The listing builds one solid part. Answer for the finished solid, in the listing's coordinates (mm). A direction names the side the tool comes from. Give positions to 0.01 mm unless a question says otherwise; leave off trailing zeros. Order: outer loops, then holes, each group sorted by start corner. A loop starts at its lowest first (then second) coordinate and runs counter-clockwise, first axis right, second up. Notation, with made-up numbers: (5.5, 69) - (48.5, 69) arc R14 cw to (48.5, 82) - close; hole circle Ø8 at (-38.75, 33.25). An arc over 180 degrees is marked (long way). Answer in a Markdown table with one row per item. Add a question column.
```python
from build123d import *

# Parameters (mm, degrees)
SKETCH2_W           = 165
SKETCH2_H           = 140
SKETCH2_W_2         = 3
SKETCH2_H_2         = 146.3
SKETCH2_W_3         = 2.5
BOSS_EXTRUDE1_DEPTH = 5
SKETCH2_3_R         = 1.7
BOSS_EXTRUDE2_DEPTH = 2.5
SKETCH2_5_R         = 4
SKETCH2_5_R_2       = 1.7
BOSS_EXTRUDE3_DEPTH = 3
FILLET1_R           = 2


with BuildPart() as part:
    # Sketch2 → Boss-Extrude1 (new body)
    with BuildSketch(Plane(origin=(0, 0, 0), x_dir=(1, 0, 0), z_dir=(0, 1, 0))):
        Polygon((-88.5, -80), (-92.5, -80), (-92.5, -78.85), (-95.5, -78.85), (-95.5, -82.5), (95, -82.5), (95, -78.85), (92.5, -78.85), (92.5, -80), (88.5, -80), align=None)
        with BuildLine():
            Line((-92.5, -78.85), (-92.5, -80))
            Line((-92.5, -80), (-88.5, -80))
            ThreePointArc((-88.5, -80), (-90.016575089, -79.701351105), (-91.30668844, -78.85))
            Line((-91.30668844, -78.85), (-92.5, -78.85))
        make_face()
        with BuildLine():
            ThreePointArc((-91.30668844, -78.85), (-90.016575089, -79.701351105), (-88.5, -80))
            ThreePointArc((-88.5, -80), (-85.671572875, -78.828427125), (-84.5, -76))
            ThreePointArc((-84.5, -76), (-86.955130064, -72.310369005), (-91.30668844, -73.15))
            Line((-91.30668844, -73.15), (-90.145448267, -73.15))
            Line((-90.145448267, -73.15), (-86.854551733, -73.15))
            Line((-86.854551733, -73.15), (-85.209103466, -76))
            Line((-85.209103466, -76), (-86.854551733, -78.85))
            Line((-86.854551733, -78.85), (-90.145448267, -78.85))
            Line((-90.145448267, -78.85), (-91.30668844, -78.85))
        make_face()
        with BuildLine():
            ThreePointArc((-84.5, -76), (-85.671572875, -78.828427125), (-88.5, -80))
            Line((-88.5, -80), (88.5, -80))
            ThreePointArc((88.5, -80), (84.798648895, -74.483424911), (91.30668844, -73.15))
            Line((91.30668844, -73.15), (92.5, -73.15))
            Line((92.5, -73.15), (92.5, 73.15))
            Line((92.5, 73.15), (91.30668844, 73.15))
            ThreePointArc((91.30668844, 73.15), (84.798648895, 74.483424911), (88.5, 80))
            Line((88.5, 80), (-88.5, 80))
            ThreePointArc((-88.5, 80), (-85.671572875, 78.828427125), (-84.5, 76))
            ThreePointArc((-84.5, 76), (-86.955130064, 72.310369005), (-91.30668844, 73.15))
            Line((-91.30668844, 73.15), (-92.5, 73.15))
            Line((-92.5, 73.15), (-92.5, -73.15))
            Line((-92.5, -73.15), (-91.30668844, -73.15))
            ThreePointArc((-91.30668844, -73.15), (-86.955130064, -72.310369005), (-84.5, -76))
        make_face()
        Rectangle(SKETCH2_W, SKETCH2_H, mode=Mode.SUBTRACT)
        with Locations((-94, 0)):
            Rectangle(SKETCH2_W_2, SKETCH2_H_2)
        with BuildLine():
            Line((-92.5, 80), (-92.5, 78.85))
            Line((-92.5, 78.85), (-91.30668844, 78.85))
            ThreePointArc((-91.30668844, 78.85), (-90.016575089, 79.701351105), (-88.5, 80))
            Line((-88.5, 80), (-92.5, 80))
        make_face()
        with BuildLine():
            Line((-90.145448267, 73.15), (-91.30668844, 73.15))
            ThreePointArc((-91.30668844, 73.15), (-86.955130064, 72.310369005), (-84.5, 76))
            ThreePointArc((-84.5, 76), (-85.671572875, 78.828427125), (-88.5, 80))
            ThreePointArc((-88.5, 80), (-90.016575089, 79.701351105), (-91.30668844, 78.85))
            Line((-91.30668844, 78.85), (-90.145448267, 78.85))
            Line((-90.145448267, 78.85), (-86.854551733, 78.85))
            Line((-86.854551733, 78.85), (-85.209103466, 76))
            Line((-85.209103466, 76), (-86.854551733, 73.15))
            Line((-86.854551733, 73.15), (-90.145448267, 73.15))
        make_face()
        with BuildLine():
            Line((91.30668844, 78.85), (92.5, 78.85))
            Line((92.5, 78.85), (92.5, 80))
            Line((92.5, 80), (88.5, 80))
            ThreePointArc((88.5, 80), (90.016575089, 79.701351105), (91.30668844, 78.85))
        make_face()
        with BuildLine():
            ThreePointArc((88.5, 80), (84.798648895, 74.483424911), (91.30668844, 73.15))
            Line((91.30668844, 73.15), (90.145448267, 73.15))
            Line((90.145448267, 73.15), (86.854551733, 73.15))
            Line((86.854551733, 73.15), (85.209103466, 76))
            Line((85.209103466, 76), (86.854551733, 78.85))
            Line((86.854551733, 78.85), (90.145448267, 78.85))
            Line((90.145448267, 78.85), (91.30668844, 78.85))
            ThreePointArc((91.30668844, 78.85), (90.016575089, 79.701351105), (88.5, 80))
        make_face()
        Polygon((-95.5, 82.5), (-95.5, 78.85), (-92.5, 78.85), (-92.5, 80), (-88.5, 80), (88.5, 80), (92.5, 80), (92.5, 78.85), (95, 78.85), (95, 82.5), align=None)
        with Locations((93.75, 0)):
            Rectangle(SKETCH2_W_3, SKETCH2_H_2)
        with BuildLine():
            ThreePointArc((91.30668844, -73.15), (84.798648895, -74.483424911), (88.5, -80))
            ThreePointArc((88.5, -80), (90.016575089, -79.701351105), (91.30668844, -78.85))
            Line((91.30668844, -78.85), (90.145448267, -78.85))
            Line((90.145448267, -78.85), (86.854551733, -78.85))
            Line((86.854551733, -78.85), (85.209103466, -76))
            Line((85.209103466, -76), (86.854551733, -73.15))
            Line((86.854551733, -73.15), (90.145448267, -73.15))
            Line((90.145448267, -73.15), (91.30668844, -73.15))
        make_face()
        with BuildLine():
            ThreePointArc((91.30668844, -78.85), (90.016575089, -79.701351105), (88.5, -80))
            Line((88.5, -80), (92.5, -80))
            Line((92.5, -80), (92.5, -78.85))
            Line((92.5, -78.85), (91.30668844, -78.85))
        make_face()
    extrude(amount=-BOSS_EXTRUDE1_DEPTH)

    # Sketch2_3 → Boss-Extrude2 (add)
    with BuildSketch(Plane(origin=(0, 0, 0), x_dir=(1, 0, 0), z_dir=(0, 1, 0))):
        Polygon((-95.5, -78.85), (-86.854551733, -78.85), (-85.209103466, -76), (-86.854551733, -73.15), (-95.5, -73.15), align=None)
        with Locations((-88.5, -76)):
            Circle(SKETCH2_3_R, mode=Mode.SUBTRACT)
        Polygon((95, -78.85), (95, -73.15), (86.854551733, -73.15), (85.209103466, -76), (86.854551733, -78.85), align=None)
        with Locations((88.5, -76)):
            Circle(SKETCH2_3_R, mode=Mode.SUBTRACT)
        Polygon((-95.5, 73.15), (-86.854551733, 73.15), (-85.209103466, 76), (-86.854551733, 78.85), (-95.5, 78.85), align=None)
        with Locations((-88.5, 76)):
            Circle(SKETCH2_3_R, mode=Mode.SUBTRACT)
        Polygon((95, 73.15), (95, 78.85), (86.854551733, 78.85), (85.209103466, 76), (86.854551733, 73.15), align=None)
        with Locations((88.5, 76)):
            Circle(SKETCH2_3_R, mode=Mode.SUBTRACT)
    extrude(amount=-BOSS_EXTRUDE2_DEPTH)

    # Sketch2_5 → Boss-Extrude3 (add)
    with BuildSketch(Plane(origin=(0, 0, 0), x_dir=(1, 0, 0), z_dir=(0, 1, 0))):
        with Locations((-88.5, -76)):
            Circle(SKETCH2_5_R)
        with Locations((-88.5, -76)):
            Circle(SKETCH2_5_R_2, mode=Mode.SUBTRACT)
        with Locations((-88.5, 76)):
            Circle(SKETCH2_5_R)
        with Locations((-88.5, 76)):
            Circle(SKETCH2_5_R_2, mode=Mode.SUBTRACT)
        with Locations((88.5, 76)):
            Circle(SKETCH2_5_R)
        with Locations((88.5, 76)):
            Circle(SKETCH2_5_R_2, mode=Mode.SUBTRACT)
        with Locations((88.5, -76)):
            Circle(SKETCH2_5_R)
        with Locations((88.5, -76)):
            Circle(SKETCH2_5_R_2, mode=Mode.SUBTRACT)
    extrude(amount=BOSS_EXTRUDE3_DEPTH)

    # Fillet1
    fillet1_edges = [part.edges().sort_by_distance(p)[0] for p in [
        (95, -2.5, 82.5),
        (-95.5, -2.5, 82.5),
        (-95.5, -2.5, -82.5),
        (95, -2.5, -82.5),
    ]]
    fillet(fillet1_edges, radius=FILLET1_R)


solid = part.part
```
(1) This flat-tipped pin is pushed along its axis until it touches: P1, Ø4, axis at x = 88.5, z = 76, coming from the -Y side. Where does it stop, or does it pass through?
(2) For faces 1 (the face through (91, -2.5, -76)), 2 (the face through (95, -2, 1)), 3 (the face through (-82.5, -2, 1)), 4 (the face through (-2, 0, 72)), 5 (the face through (-92, -2.5, -76)), determine the directions among +Z, -Z, +X, -X, +Y, -Y from which every point of the face is accessible in a straight line to the end or side of a thin tool.
(3) Straight lines are drawn through the part: line 1 (Z direction, x = -88.5, y = -1.55); line 2 (X direction, y = 1.7, z = -76); line 3 (X direction, y = -0.5, z = -34.5). For each, find the intervals that lie inside material, in ascending order.
(4) Find section C-C, the plane z = -19. Write down the section's boundary in (x, y).
(5) Find section A-A, the plane x = -35.5. Write down the section's boundary in (y, z).
(6) The mould has two halves that part along X. Classify faces 6 (the face through (-95.5, -2, -1)), 7 (the face through (-1, -2, 70)), 8 (the face through (-92, -2.5, 76)): +X half, -X half, draft (parallel to the pull), parting line (faces both ways), or undercut.
(7) Find section B-B, the plane y = 1.5. Write down the section's boundary in (x, z), plus the area to 3 significant figures.
Answer key:
| question | item | result |
|---|---|---|
| 1 | P1 | y = -2.5 |
| 2 | face 1 | +X, -Y |
| 2 | face 2 | +Z, -Z, +X, +Y, -Y |
| 2 | face 3 | +Y, -Y |
| 2 | face 4 | +Y |
| 2 | face 5 | -X, -Y |
| 3 | line 1 | -82.5 to -77.7, -74.3 to 74.3, 77.7 to 82.5 |
| 3 | line 2 | -92.5 to -90.2, -86.8 to -84.5, 84.5 to 86.8, 90.2 to 92.5 |
| 3 | line 3 | -95.5 to -82.5, 82.5 to 95 |
| 4 | outline | (-95.5, -5) - (-82.5, -5) - (-82.5, 0) - (-95.5, 0) - close; (82.5, -5) - (95, -5) - (95, 0) - (82.5, 0) - close |
| 5 | outline | (-5, -82.5) - (0, -82.5) - (0, -70) - (-5, -70) - close; (-5, 70) - (0, 70) - (0, 82.5) - (-5, 82.5) - close |
| 6 | face 6 | -X half |
| 6 | face 7 | undercut |
| 6 | face 8 | draft |
| 7 | outline | circle Ø8 at (-88.5, -76); circle Ø8 at (-88.5, 76); circle Ø8 at (88.5, -76); circle Ø8 at (88.5, 76); hole circle Ø3.4 at (-88.5, -76); hole circle Ø3.4 at (-88.5, 76); hole circle Ø3.4 at (88.5, -76); hole circle Ø3.4 at (88.5, 76) |
| 7 | area | 165 mm² |
